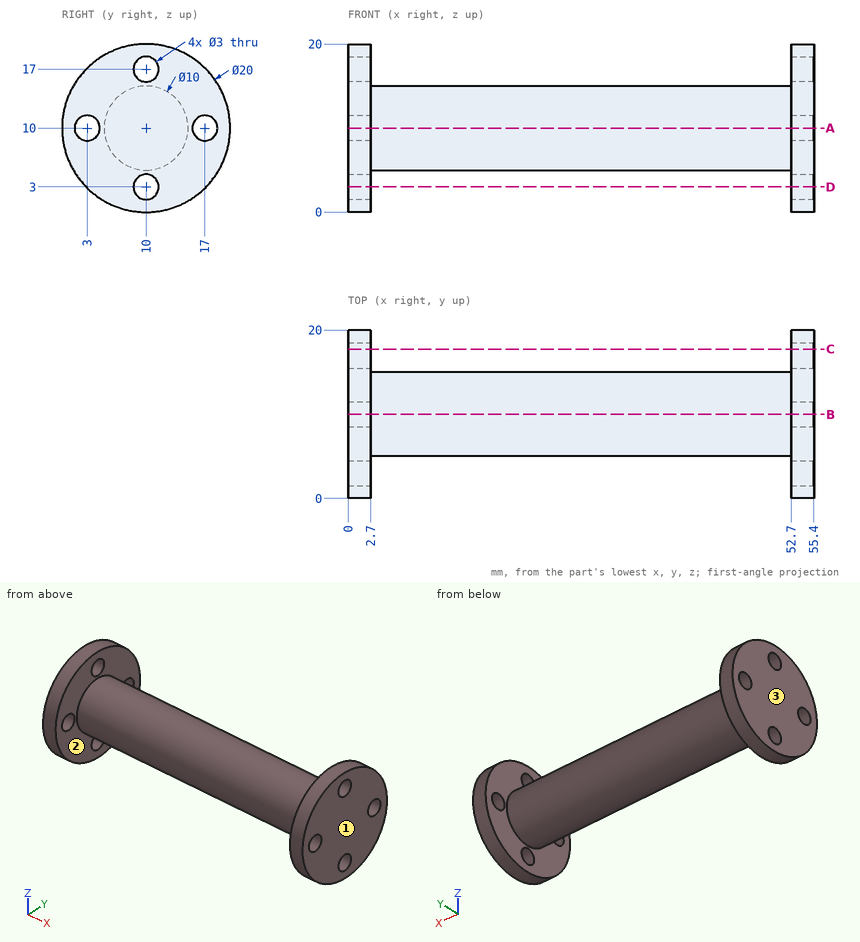
Verification items for this drawing (mm, ordinates from the low corner). Coordinates: 2 decimals unless noted, no trailing zeros. Order: outer loops, then holes, each group sorted by start corner. A loop starts at its lowest first (then second) coordinate and runs counter-clockwise, first axis right, second up. Notation, with made-up numbers: (89.5, 0.5) - (119.5, 0.5) arc R24 ccw to (119.5, 39.5) - close; hole circle Ø5 at (68, 63). An arc over 180 degrees is marked (long way). Answer in a Markdown table with one row per item. Add a question column.
1. Section check D-D (z = 3). Enter the section's corners in (x, y), plus the area to 3 significant figures.
2. Gauge pin test, flat ends, axial feed: pin 1 Ø1.8 at (y, z) = (10, 3) entering from +X; pin 2 Ø1 at (x, y) = (15, 13.5) entering from +Z; pin 3 Ø5 at (x, z) = (37.5, 16.5) entering from -Y; pin 4 Ø3 at (x, z) = (11.5, 5.5) entering from -Y. Record the tip position at first contact, or that the pin passes through.
3. Material ranges on L1, parallel to X at y = 1.25, z = 11.75; L2, parallel to Y at x = 1.45, z = 10; L3, parallel to Y at x = 54.1, z = 3, recorded low to high. Write a range as [from, to].
4. Section check A-A (z = 10). Enter the section's corners in (x, y).
5. Section check C-C (y = 17.75). Enter the section's corners in (x, z), plus the area to 3 significant figures.
6. Draft check along X on the marked faces 1, 2 and 3. Enter one of: +X half, -X half, draft (parallel to the pull), parting line (faces both ways), or undercut.
Data:
| question | item | result |
|---|---|---|
| 1 | outline | (0, 2.86) - (2.7, 2.86) - (2.7, 8.5) - (0, 8.5) - close; (0, 11.5) - (2.7, 11.5) - (2.7, 17.14) - (0, 17.14) - close; (52.7, 2.86) - (55.4, 2.86) - (55.4, 8.5) - (52.7, 8.5) - close; (52.7, 11.5) - (55.4, 11.5) - (55.4, 17.14) - (52.7, 17.14) - close |
| 1 | area | 60.9 mm² |
| 2 | pin 1 | passes through |
| 2 | pin 2 | stops at z = 14 |
| 2 | pin 3 | stops at y = 7 |
| 2 | pin 4 | stops at y = 6 |
| 3 | L1 | x = [0, 2.7], [52.7, 55.4] |
| 3 | L2 | y = [0, 1.5], [4.5, 15.5], [18.5, 20] |
| 3 | L3 | y = [2.86, 8.5], [11.5, 17.14] |
| 4 | outline | (0, 0) - (2.7, 0) - (2.7, 1.5) - (0, 1.5) - close; (0, 4.5) - (2.7, 4.5) - (2.7, 5) - (52.7, 5) - (52.7, 4.5) - (55.4, 4.5) - (55.4, 15.5) - (52.7, 15.5) - (52.7, 15) - (2.7, 15) - (2.7, 15.5) - (0, 15.5) - close; (0, 18.5) - (2.7, 18.5) - (2.7, 20) - (0, 20) - close; (52.7, 0) - (55.4, 0) - (55.4, 1.5) - (52.7, 1.5) - close; (52.7, 18.5) - (55.4, 18.5) - (55.4, 20) - (52.7, 20) - close |
| 5 | outline | (0, 3.68) - (2.7, 3.68) - (2.7, 8.7) - (0, 8.7) - close; (0, 11.3) - (2.7, 11.3) - (2.7, 16.32) - (0, 16.32) - close; (52.7, 3.68) - (55.4, 3.68) - (55.4, 8.7) - (52.7, 8.7) - close; (52.7, 11.3) - (55.4, 11.3) - (55.4, 16.32) - (52.7, 16.32) - close |
| 5 | area | 54.2 mm² |
| 6 | face 1 | +X half |
| 6 | face 2 | undercut |
| 6 | face 3 | -X half |
